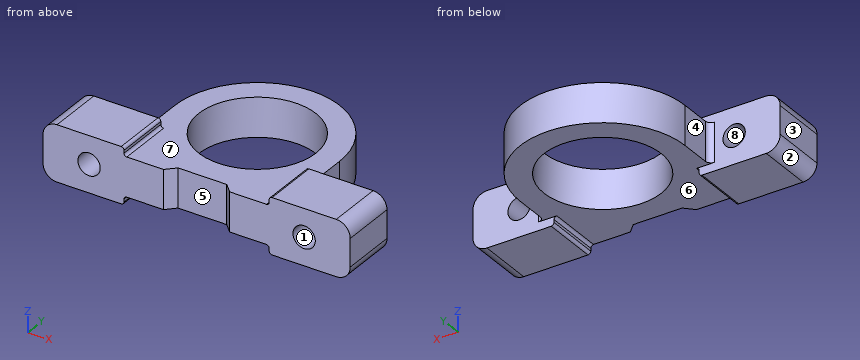
from build123d import *

# Parameters (mm, degrees)
SKETCH1_R           = 21
BOSS_EXTRUDE1_DEPTH = 7
SKETCH2_W           = 29
SKETCH2_H           = 20
BOSS_EXTRUDE2_DEPTH = 3
CUT_EXTRUDE1_DEPTH  = 67.355105305
FILLET1_R           = 5
FILLET2_R           = 1
SKETCH4_R           = 4
CUT_EXTRUDE2_DEPTH  = 71.222859526


with BuildPart() as part:
    # Sketch1 → Boss-Extrude1 (new, symmetric)
    with BuildSketch(Plane.XY):
        with BuildLine():
            Line((-29.5, 0), (-29.5, -11))
            ThreePointArc((-29.5, -11), (-30.085786438, -12.414213562), (-31.5, -13))
            Line((-31.5, -13), (-55, -13))
            Line((-55, -13), (-55, -33))
            Line((-55, -33), (55, -33))
            Line((55, -33), (55, -13))
            Line((55, -13), (31.5, -13))
            ThreePointArc((31.5, -13), (30.085786438, -12.414213562), (29.5, -11))
            Line((29.5, -11), (29.5, 0))
            ThreePointArc((29.5, 0), (0, 29.5), (-29.5, 0))
        make_face()
        Circle(SKETCH1_R, mode=Mode.SUBTRACT)
    extrude(amount=BOSS_EXTRUDE1_DEPTH, both=True)

    # Sketch2 → Boss-Extrude2 (add)
    with BuildSketch(Plane.XY.offset(7)):
        with Locations((-40.5, -23)):
            Rectangle(SKETCH2_W, SKETCH2_H)
        with Locations((40.5, -23)):
            Rectangle(SKETCH2_W, SKETCH2_H)
    boss_extrude2 = extrude(amount=BOSS_EXTRUDE2_DEPTH)

    # Mirror1: Boss-Extrude2 across plane
    add(boss_extrude2.mirror(Plane.XY))

    # Sketch3 → Cut-Extrude1 (cut, through all)
    with BuildSketch(Plane.XY.offset(7)):
        Polygon((-11.85382749, -33), (-8.732636014, -29.878808524), (8.732636014, -29.878808524), (11.85382749, -33), align=None)
    extrude(amount=-CUT_EXTRUDE1_DEPTH, mode=Mode.SUBTRACT)

    # Fillet1
    fillet1_edges = [part.edges().sort_by_distance(p)[0] for p in [
        (-55, -23, 10),
        (55, -23, 10),
        (-55, -23, -10),
        (55, -23, -10),
    ]]
    fillet(fillet1_edges, radius=FILLET1_R)

    # Fillet2
    fillet2_edges = [part.edges().sort_by_distance(p)[0] for p in [
        (-26, -23, 7),
        (-26, -23, 10),
        (26, -23, 7),
        (26, -23, 10),
        (-26, -23, -10),
        (-26, -23, -7),
        (26, -23, -10),
        (26, -23, -7),
    ]]
    fillet(fillet2_edges, radius=FILLET2_R)

    # Sketch4 → Cut-Extrude2 (cut, through all)
    with BuildSketch(Plane(origin=(0, -13, 0), x_dir=(1, 0, 0), z_dir=(0, 1, 0))):
        with Locations(Location((38.5, 0, 0), (0, 0, 180))):
            Circle(SKETCH4_R)
        with Locations((-38.5, 0)):
            Circle(SKETCH4_R)
    extrude(amount=-CUT_EXTRUDE2_DEPTH, mode=Mode.SUBTRACT)


solid = part.part
The listing builds one solid part. Answer for the finished solid, in the listing's coordinates (mm). Face numbers are marked on the shaded views. A direction names the side the tool comes from. Give positions to 0.01 mm unless a question says otherwise; leave off trailing zeros. Loops run counter-clockwise (first coordinate to the right, second up) from the corner with the lowest first, then second, coordinate; pieces in that order, holes last.
Item 1: Determine the mould class of the marked faces 1, 2 and 3 for opening direction Z: +Z half, -Z half, draft (parallel to the pull), parting line (faces both ways), or undercut.
Derived:
face 1: undercut
face 2: -Z half
face 3: draft
Item 2: A cutting plane is placed at D-D (y = 2). Give the vertices of the cut face in (x, z).
Derived:
outline: (-29.43, -7) - (-20.9, -7) - (-20.9, 7) - (-29.43, 7) - close; (20.9, -7) - (29.43, -7) - (29.43, 7) - (20.9, 7) - close
Item 3: A cutting plane is placed at C-C (y = -18). Give the number of separate pieces and of enclosed holes in the cut face, then the cut area to 3 significant figures.
Derived:
separate pieces: 2
enclosed holes: 2
area: 1,460 mm2
Item 4: Each of these flat-tipped pins is pushed along its axis until it touches: pin 1 Ø3 at (x, z) = (6.5, -4) entering from +Y; pin 2 Ø1.1 at (y, z) = (-23.5, 8.5) entering from +X; pin 3 Ø12 at (x, y) = (-8.5, -16.5) entering from -Z. Where does it stop, or does it pass through?
Derived:
pin 1: stops at y = 29.07
pin 2: stops at x = 54.04
pin 3: stops at z = -7
Item 5: Find the intervals of material crossed by line 1 along Y through (x, z) = (0.5, 5); line 2 along Z through (x, y) = (38.5, -21.75); line 3 along X through (y, z) = (-29.5, 1.5), in increasing order.
Derived:
line 1: y = -29.88 to -20.99, 20.99 to 29.5
line 2: z = -10 to -4, 4 to 10
line 3: x = -55 to -42.21, -34.79 to 34.79, 42.21 to 55
Item 6: A cutting plane is placed at A-A (z = 0). Give the vertices of the cut face in (x, y), then the cut area to 3 significant figures.
Derived:
outline: (-55, -33) - (-42.5, -33) - (-42.5, -13) - (-55, -13) - close; (-34.5, -33) - (-11.85, -33) - (-8.73, -29.88) - (8.73, -29.88) - (11.85, -33) - (34.5, -33) - (34.5, -13) - (31.5, -13) arc R2 cw to (29.5, -11) - (29.5, 0) arc R29.5 ccw to (-29.5, 0) - (-29.5, -11) arc R2 cw to (-31.5, -13) - (-34.5, -13) - close; (42.5, -33) - (55, -33) - (55, -13) - (42.5, -13) - close; hole circle Ø42 at (0, 0)
area: 2,570 mm2
Item 7: A cutting plane is placed at B-B (x = 38.5). Give the vertices of the cut face in (y, z).
Derived:
outline: (-33, -10) - (-13, -10) - (-13, -4) - (-33, -4) - close; (-33, 4) - (-13, 4) - (-13, 10) - (-33, 10) - close
Item 8: A tool of negligible diameter and unlimited length cuts with its end or side. For the marked faces 4, 5, 6, 7 and 8, from which of +Z, -Z, +X, -X, +Y, -Y can it reach the whole face along a straight path? Write none if from no direction.
Derived:
face 4: +Z, -Z, -X, +Y
face 5: +Z, -Z, -Y
face 6: -Z, +Y
face 7: +Z, +Y
face 8: +Y, -Y
